The model under review builds one solid part; all positions refer to its coordinate system, in mm. Face numbers are marked on the shaded views. Give positions to 0.01 mm unless a question says otherwise; leave off trailing zeros. Order: outer loops, then holes, each group sorted by start corner. A loop starts at its lowest first (then second) coordinate and runs counter-clockwise, first axis right, second up. Notation, with made-up numbers: (89, 44.5) -> (98, 44.5) arc R30 ccw to (98, 69.5) -> close; hole circle Ø6 at (87, 6). An arc over 180 degrees is marked (long way). Use one line per item in the form item = value.
```python
from build123d import *

# Parameters (mm, degrees)
ESQUISSE1_R             = 3
BASE_EXTRUSION_DEPTH    = 2.5
ESQUISSE2_R             = 1.5
BOSS_EXTRU_1_DEPTH      = 22
CONG_1_R                = 0.5
ENL_V_MAT_EXTRU_1_DEPTH = 2


with BuildPart() as part:
    # Esquisse1 → Base-Extrusion (new body)
    with BuildSketch(Plane.XY):
        Circle(ESQUISSE1_R)
    extrude(amount=BASE_EXTRUSION_DEPTH)

    # Esquisse2 → Boss.-Extru.1 (add)
    with BuildSketch(Plane.XY.offset(2.5)):
        Circle(ESQUISSE2_R)
    extrude(amount=BOSS_EXTRU_1_DEPTH)

    # Congé1
    cong_1_edges = [part.edges().sort_by_distance(p)[0] for p in [
        (-3, 0, 0),
    ]]
    fillet(cong_1_edges, radius=CONG_1_R)

    # Esquisse3 → Enlèv. mat.-Extru.1 (cut)
    with BuildSketch(Plane(origin=(0, 0, 0), x_dir=(-1, 0, 0), z_dir=(0, 0, -1))):
        Polygon((1.732050808, 0), (0.866025404, 1.5), (-0.866025404, 1.5), (-1.732050808, 0), (-0.866025404, -1.5), (0.866025404, -1.5), align=None)
    extrude(amount=-ENL_V_MAT_EXTRU_1_DEPTH, mode=Mode.SUBTRACT)


solid = part.part
```
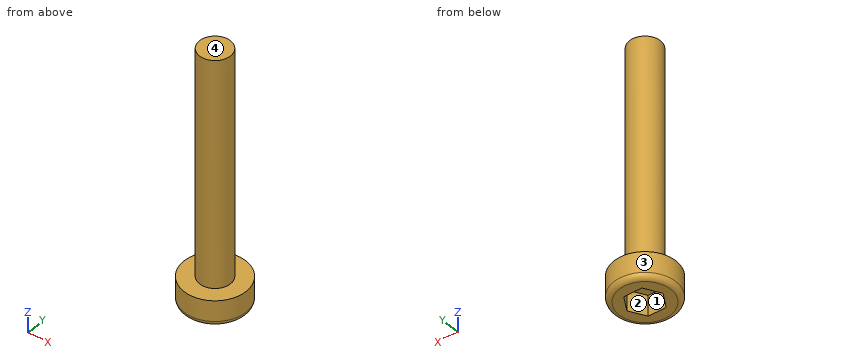
1. Add section A-A on x = 0. Give the boundary of the cut face in (y, z).
Values:
outline = (-3, 0.5) arc R0.5 ccw to (-2.5, 0) -> (-1.5, 0) -> (-1.5, 2) -> (1.5, 2) -> (1.5, 0) -> (2.5, 0) arc R0.5 ccw to (3, 0.5) -> (3, 2.5) -> (1.5, 2.5) -> (1.5, 24.5) -> (-1.5, 24.5) -> (-1.5, 2.5) -> (-3, 2.5) -> close
2. Add section B-B on z = 5. Give the boundary of the cut face in (x, y), then the cut area to 3 significant figures.
Values:
outline = circle Ø3 at (0, 0)
area = 7.07 mm^2
3. For L1, parallel to Z at x = 1.85, y = -0.55; L2, parallel to Z at x = 0.8, y = 1.1; L3, parallel to Y at x = -0.8, z = 22.75, list the stretches that pass through material, from the lowest coordinate up.
Values:
L1 = 0 to 2.5
L2 = 2 to 24.5
L3 = -1.27 to 1.27
4. For pin 1 Ø2 at (x, z) = (-1, 7.5) entering from -Y; pin 2 Ø2 at (x, y) = (-1.5, -0.5) entering from +Z; pin 3 Ø0.5 at (x, z) = (0.5, 1.5) entering from +Y; pin 4 Ø0.9 at (x, y) = (0.5, 0) entering from -Z, all flat-tipped, find the tip position at first contact; note any pin that passes through.
Values:
pin_1 = -1.5
pin_2 = 24.5
pin_3 = 2.99
pin_4 = 2
5. The part is to be moulded in two halves that separate along Y. For the marked faces 1, 2, 3 and 4, say which applies: +Y half, -Y half, draft (parallel to the pull), parting line (faces both ways), or undercut.
Values:
face_1 = undercut
face_2 = undercut
face_3 = parting line
face_4 = draft
